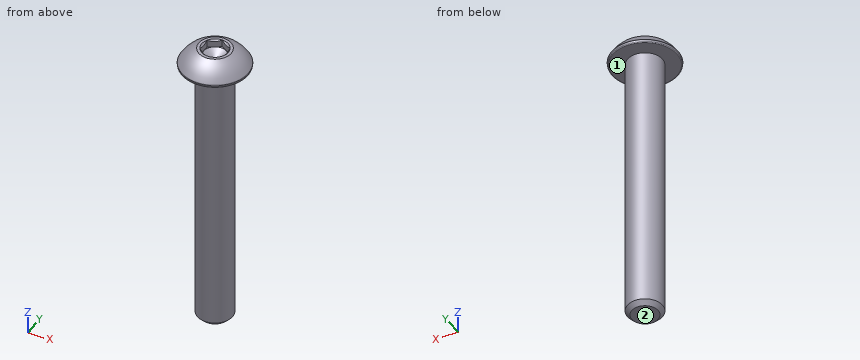
```python
from build123d import *

# Parameters (mm, degrees)
CUT_EXTRUDE1_START = 19.30654
CUT_EXTRUDE1_DEPTH = 2.02616
SKETCH4_R          = 1.833087105
CUT_EXTRUDE2_DEPTH = 1.02616
CUT_EXTRUDE2_DRAFT = -45
FILLET1_R          = 0.12827


with BuildPart() as part:
    # Sketch2 → Revolve1 (revolve)
    with BuildSketch(Plane(origin=(0, 0, 0), x_dir=(0, 0, -1), z_dir=(1, 0, 0))):
        with BuildLine():
            Line((-20.3327, 1.5875), (-20.3327, 2.2225))
            ThreePointArc((-20.3327, 2.2225), (-19.417752118, 3.57733025), (-18.130157143, 4.5847))
            Line((-18.130157143, 4.5847), (-17.7673, 4.520718496))
            Line((-17.7673, 4.520718496), (-17.7673, 2.413))
            Line((-17.7673, 2.413), (19.7373875, 2.413))
            Line((19.7373875, 2.413), (20.3327, 1.8176875))
            Line((20.3327, 1.8176875), (20.3327, 0))
            Line((20.3327, 0), (-18.389996448, 0))
            Line((-18.389996448, 0), (-19.30654, 1.5875))
            Line((-19.30654, 1.5875), (-20.3327, 1.5875))
        make_face()
    revolve(axis=Axis((0, 0, 20.3327), (0, 0, -1)))

    # Sketch3 → Cut-Extrude1 (cut, through all)
    with BuildSketch(Plane.XY.offset(CUT_EXTRUDE1_START)):
        Polygon((0, 1.833087105), (-1.5875, 0.916543552), (-1.5875, -0.916543552), (0, -1.833087105), (1.5875, -0.916543552), (1.5875, 0.916543552), align=None)
    extrude(amount=CUT_EXTRUDE1_DEPTH, mode=Mode.SUBTRACT)


with BuildPart() as cut_extrude2_tool:
    # Sketch4 → Cut-Extrude2 (with draft: the straight prism first)
    with BuildSketch(Plane.XY.offset(20.3327)):
        Circle(SKETCH4_R)
    extrude(amount=-CUT_EXTRUDE2_DEPTH)
    # Cut-Extrude2: the draft: its side faces are tilted about the plane it starts from
    cut_extrude2_sides = [cut_extrude2_tool.faces().sort_by_distance(p)[0] for p in [
        (-1.833087105, 0, 19.81962),
    ]]
    draft(cut_extrude2_sides, Plane.XY.offset(20.3327), CUT_EXTRUDE2_DRAFT)


with BuildPart() as part_1:
    add(part.part)

    # Cut-Extrude2: cut by cut_extrude2_tool
    add(cut_extrude2_tool.part, mode=Mode.SUBTRACT)

    # Fillet1
    fillet1_edges = [part_1.edges().sort_by_distance(p)[0] for p in [
        (0, -4.520718496, 17.7673),
        (0, -4.5847, 18.130157143),
    ]]
    fillet(fillet1_edges, radius=FILLET1_R)


solid = part_1.part
```
Can you work these out from the model? Positions are in its coordinate system, mm. Face numbers are marked on the shaded views. A direction names the side the tool comes from. Coordinates: 2 decimals unless noted, no trailing zeros. Loops run counter-clockwise (first coordinate to the right, second up) from the corner with the lowest first, then second, coordinate; pieces in that order, holes last.
1) Imagine slicing it at A-A on z = 14.5. List the corners of the cut face in (x, y) for me, plus the area to 3 significant figures.
2) For pin 1 (0.5 mm diameter, centred on y = -0.5, z = 19.5, fed in from -X); pin 2 (0.6 mm diameter, centred on x = 1.5, y = 0.5, fed in from +Z); pin 3 (4 mm diameter, centred on y = 1.5, z = 6.5, fed in from +X); pin 4 (1.5 mm diameter, centred on y = 2.5, z = 12.5, fed in from +X), each with a flat end and sliding along its axis, tell me the tip position at first contact or that it passes through.
3) Which directions (+Z, -Z, +X, -X, +Y, -Y) give clear straight access to the entire face, cutting with the end or side of a thin tool? Please do the marked faces 1 and 2.
4) I need wall thicknesses on probe 1 along X at (y, z) = (0, 0.5); probe 2 along Z at (x, y) = (-3.5, 2.75); probe 3 along Z at (x, y) = (-2, 2). Which ranges of each line are inside material? Lowest first, please.
Completed:
1. outline: circle Ø4.83 at (0, 0)
1. area: 18.3 mm2
2. pin 1: stops at x = -3.72
2. pin 2: stops at z = 20.33
2. pin 3: stops at x = 2.41
2. pin 4: stops at x = 1.66
3. face 1: -Z
3. face 2: -Z, +X, -X, +Y, -Y
4. probe 1: x = -2.41 to 2.41
4. probe 2: z = 17.77 to 18.36
4. probe 3: z = 17.77 to 20
